from build123d import *

# Parameters (mm, degrees)
BOSS_EXTRUDE1_DEPTH            = 64
BOSS_EXTRUDE2_DEPTH            = 12
SKETCH3_W                      = 12.5
SKETCH3_H                      = 12.5
CUT_EXTRUDE1_DEPTH             = 29
CUT_EXTRUDE2_REACH             = 106.125
SKETCH5_W                      = 12.5
SKETCH5_H                      = 17
CUT_EXTRUDE2_DIRECTION_2_REACH = 106.125
CUT_EXTRUDE3_REACH             = 116.092
SKETCH6_R                      = 2
SKETCH7_W                      = 80
SKETCH7_H                      = 29
BOSS_EXTRUDE3_DEPTH            = 10
SKETCH8_W                      = 5
SKETCH8_H                      = 17
CUT_EXTRUDE4_DEPTH             = 80


with BuildPart() as part:
    # Sketch1 → Boss-Extrude1 (new body)
    with BuildSketch(Plane.XY):
        with BuildLine():
            Line((0, 0), (80, 0))
            Line((80, 0), (80, 5))
            Line((80, 5), (71, 5))
            Line((71, 5), (71, 22))
            Line((71, 22), (80, 22))
            Line((80, 22), (80, 29))
            Line((80, 29), (65, 29))
            ThreePointArc((65, 29), (40, 4), (15, 29))
            Line((15, 29), (0, 29))
            Line((0, 29), (0, 22))
            Line((0, 22), (9, 22))
            Line((9, 22), (9, 5))
            Line((9, 5), (0, 5))
            Line((0, 5), (0, 0))
        make_face()
    extrude(amount=BOSS_EXTRUDE1_DEPTH)

    # Sketch2 → Boss-Extrude2 (add)
    with BuildSketch(Plane.XY.offset(64)):
        with BuildLine():
            Line((60, 29), (80, 29))
            Line((80, 29), (80, 0))
            Line((80, 0), (0, 0))
            Line((0, 0), (0, 29))
            Line((0, 29), (20, 29))
            ThreePointArc((20, 29), (40, 9), (60, 29))
        make_face()
    extrude(amount=BOSS_EXTRUDE2_DEPTH)

    # Sketch3 → Cut-Extrude1 (cut)
    with BuildSketch(Plane(origin=(0, 29, 0), x_dir=(1, 0, 0), z_dir=(0, 1, 0))):
        with Locations((21.25, -16)):
            Rectangle(SKETCH3_W, SKETCH3_H)
        with Locations((58.75, -16)):
            Rectangle(SKETCH3_W, SKETCH3_H)
        with Locations((21.25, -48)):
            Rectangle(SKETCH3_W, SKETCH3_H)
        with Locations((58.75, -48)):
            Rectangle(SKETCH3_W, SKETCH3_H)
    extrude(amount=-CUT_EXTRUDE1_DEPTH, mode=Mode.SUBTRACT)

    # Cut-Extrude2: up to this face of the body (flat: up to its plane)
    cut_extrude2_end = Plane(part.part.faces().sort_by_distance((9, 13.5, 32))[0])
    # Sketch5 → Cut-Extrude2 (cut, up to the picked face)
    with BuildSketch(Plane(origin=(15, 0, 0), x_dir=(0, 0, -1), z_dir=(1, 0, 0)), mode=Mode.PRIVATE) as cut_extrude2_sk1:
        with Locations((-48, 13.5)):
            Rectangle(SKETCH5_W, SKETCH5_H)
    cut_extrude2_tool1 = split(extrude(cut_extrude2_sk1.sketch, amount=-CUT_EXTRUDE2_REACH, mode=Mode.PRIVATE), bisect_by=cut_extrude2_end, keep=Keep.BOTH, mode=Mode.PRIVATE)
    # Sketch5 → Cut-Extrude2 (cut, up to the picked face)
    with BuildSketch(Plane(origin=(15, 0, 0), x_dir=(0, 0, -1), z_dir=(1, 0, 0)), mode=Mode.PRIVATE) as cut_extrude2_sk2:
        with Locations((-16, 13.5)):
            Rectangle(SKETCH5_W, SKETCH5_H)
    cut_extrude2_tool2 = split(extrude(cut_extrude2_sk2.sketch, amount=-CUT_EXTRUDE2_REACH, mode=Mode.PRIVATE), bisect_by=cut_extrude2_end, keep=Keep.BOTH, mode=Mode.PRIVATE)
    add(cut_extrude2_tool1.solids().sort_by(Axis((15, 13.5, 48), (-1, 0, 0)))[0], mode=Mode.SUBTRACT)
    add(cut_extrude2_tool2.solids().sort_by(Axis((15, 13.5, 16), (-1, 0, 0)))[0], mode=Mode.SUBTRACT)

    # Cut-Extrude2 direction 2: up to this face of the body (flat: up to its plane)
    cut_extrude2_direction_2_end = Plane(part.part.faces().sort_by_distance((71, 13.5, 32))[0])
    # Sketch5 → Cut-Extrude2 direction 2 (cut, up to the picked face)
    with BuildSketch(Plane(origin=(15, 0, 0), x_dir=(0, 0, -1), z_dir=(1, 0, 0)), mode=Mode.PRIVATE) as cut_extrude2_direction_2_sk1:
        with Locations((-48, 13.5)):
            Rectangle(SKETCH5_W, SKETCH5_H)
    cut_extrude2_direction_2_tool1 = split(extrude(cut_extrude2_direction_2_sk1.sketch, amount=CUT_EXTRUDE2_DIRECTION_2_REACH, mode=Mode.PRIVATE), bisect_by=cut_extrude2_direction_2_end, keep=Keep.BOTH, mode=Mode.PRIVATE)
    # Sketch5 → Cut-Extrude2 direction 2 (cut, up to the picked face)
    with BuildSketch(Plane(origin=(15, 0, 0), x_dir=(0, 0, -1), z_dir=(1, 0, 0)), mode=Mode.PRIVATE) as cut_extrude2_direction_2_sk2:
        with Locations((-16, 13.5)):
            Rectangle(SKETCH5_W, SKETCH5_H)
    cut_extrude2_direction_2_tool2 = split(extrude(cut_extrude2_direction_2_sk2.sketch, amount=CUT_EXTRUDE2_DIRECTION_2_REACH, mode=Mode.PRIVATE), bisect_by=cut_extrude2_direction_2_end, keep=Keep.BOTH, mode=Mode.PRIVATE)
    add(cut_extrude2_direction_2_tool1.solids().sort_by(Axis((15, 13.5, 48), (1, 0, 0)))[0], mode=Mode.SUBTRACT)
    add(cut_extrude2_direction_2_tool2.solids().sort_by(Axis((15, 13.5, 16), (1, 0, 0)))[0], mode=Mode.SUBTRACT)

    # Cut-Extrude3: up to this face of the body (flat: up to its plane)
    cut_extrude3_end = Plane(part.part.faces().sort_by_distance((72, 29, 39.6))[0])
    # Sketch6 → Cut-Extrude3 (cut, up to the picked face)
    with BuildSketch(Plane(origin=(0, 0, 0), x_dir=(-1, 0, 0), z_dir=(0, -1, 0)), mode=Mode.PRIVATE) as cut_extrude3_sk1:
        with Locations(Location((-4.499910861, -59.125, 0), (0, 0, 90))):
            Circle(SKETCH6_R)
    cut_extrude3_tool1 = split(extrude(cut_extrude3_sk1.sketch, amount=-CUT_EXTRUDE3_REACH, mode=Mode.PRIVATE), bisect_by=cut_extrude3_end, keep=Keep.BOTH, mode=Mode.PRIVATE)
    # Sketch6 → Cut-Extrude3 (cut, up to the picked face)
    with BuildSketch(Plane(origin=(0, 0, 0), x_dir=(-1, 0, 0), z_dir=(0, -1, 0)), mode=Mode.PRIVATE) as cut_extrude3_sk2:
        with Locations(Location((-4.499910861, -4.875, 0), (0, 0, 180))):
            Circle(SKETCH6_R)
    cut_extrude3_tool2 = split(extrude(cut_extrude3_sk2.sketch, amount=-CUT_EXTRUDE3_REACH, mode=Mode.PRIVATE), bisect_by=cut_extrude3_end, keep=Keep.BOTH, mode=Mode.PRIVATE)
    # Sketch6 → Cut-Extrude3 (cut, up to the picked face)
    with BuildSketch(Plane(origin=(0, 0, 0), x_dir=(-1, 0, 0), z_dir=(0, -1, 0)), mode=Mode.PRIVATE) as cut_extrude3_sk3:
        with Locations(Location((-75.500089139, -4.875, 0), (0, 0, 180))):
            Circle(SKETCH6_R)
    cut_extrude3_tool3 = split(extrude(cut_extrude3_sk3.sketch, amount=-CUT_EXTRUDE3_REACH, mode=Mode.PRIVATE), bisect_by=cut_extrude3_end, keep=Keep.BOTH, mode=Mode.PRIVATE)
    # Sketch6 → Cut-Extrude3 (cut, up to the picked face)
    with BuildSketch(Plane(origin=(0, 0, 0), x_dir=(-1, 0, 0), z_dir=(0, -1, 0)), mode=Mode.PRIVATE) as cut_extrude3_sk4:
        with Locations(Location((-75.500089139, -59.125, 0), (0, 0, 180))):
            Circle(SKETCH6_R)
    cut_extrude3_tool4 = split(extrude(cut_extrude3_sk4.sketch, amount=-CUT_EXTRUDE3_REACH, mode=Mode.PRIVATE), bisect_by=cut_extrude3_end, keep=Keep.BOTH, mode=Mode.PRIVATE)
    add(cut_extrude3_tool1.solids().sort_by(Axis((4.499911, 0, 59.125), (0, 1, 0)))[0], mode=Mode.SUBTRACT)
    add(cut_extrude3_tool2.solids().sort_by(Axis((4.499911, 0, 4.875), (0, 1, 0)))[0], mode=Mode.SUBTRACT)
    add(cut_extrude3_tool3.solids().sort_by(Axis((75.500089, 0, 4.875), (0, 1, 0)))[0], mode=Mode.SUBTRACT)
    add(cut_extrude3_tool4.solids().sort_by(Axis((75.500089, 0, 59.125), (0, 1, 0)))[0], mode=Mode.SUBTRACT)

    # Sketch7 → Boss-Extrude3 (add)
    with BuildSketch(Plane(origin=(0, 0, 0), x_dir=(-1, 0, 0), z_dir=(0, 0, -1))):
        with Locations((-40, 14.5)):
            Rectangle(SKETCH7_W, SKETCH7_H)
    extrude(amount=BOSS_EXTRUDE3_DEPTH)

    # Sketch8 → Cut-Extrude4 (cut)
    with BuildSketch(Plane(origin=(80, 0, 0), x_dir=(0, 0, -1), z_dir=(1, 0, 0))):
        with Locations((2.5, 13.5)):
            Rectangle(SKETCH8_W, SKETCH8_H)
    extrude(amount=-CUT_EXTRUDE4_DEPTH, mode=Mode.SUBTRACT)


solid = part.part
Work out the finished part from the listing and answer in its coordinate system (mm). A direction names the side the tool comes from. Give positions to 0.01 mm unless a question says otherwise; leave off trailing zeros. Write each loop counter-clockwise with the first axis right and the second up, starting at its lowest first coordinate (ties: lowest second). Pieces come first, ordered by that corner, then holes.
Q1. The part is cut by section C-C on x = 40. Give the vertices of the cut face in (y, z), and give its area (3 significant figures).
Answer:
outline: (0, -10) - (29, -10) - (29, 0) - (22, 0) - (22, -5) - (5, -5) - (5, 0) - (4, 0) - (4, 64) - (9, 64) - (9, 76) - (0, 76) - close
area: 569 mm2
Q2. The part is cut by section B-B on x = 25.5. Give the vertices of the cut face in (y, z).
Answer:
outline: (0, -10) - (29, -10) - (29, 0) - (22, 0) - (22, -5) - (5, -5) - (5, 0) - (8.63, 0) - (8.63, 9.75) - (0, 9.75) - close; (0, 22.25) - (8.63, 22.25) - (8.63, 41.75) - (0, 41.75) - close; (0, 54.25) - (8.63, 54.25) - (8.63, 64) - (15.23, 64) - (15.23, 76) - (0, 76) - close
Q3. Straight lines are drawn through the part: L1, parallel to Z at x = 15, y = 15.25; L2, parallel to Z at x = 18, y = 3.25; L3, parallel to Y at x = 5, z = 31. For each, find the intervals that lie inside material, in ascending order.
Answer:
L1: z = -10 to -5, 0 to 9.75, 22.25 to 41.75, 54.25 to 76
L2: z = -10 to 9.75, 22.25 to 41.75, 54.25 to 76
L3: y = 0 to 5, 22 to 29
Q4. Given pin 1 (7.5 mm diameter, centred on x = 34.5, y = 26.5, fed in from +Z); pin 2 (8 mm diameter, centred on y = 17.5, z = 25.5, fed in from +X); pin 3 (5 mm diameter, centred on y = 17, z = 7, fed in from -X), each flat-ended and moving along its own axis, determine where each tip first touches the part or whether it passes through.
Answer:
pin 1: stops at z = 0
pin 2: stops at x = 71
pin 3: stops at x = 9
Q5. A tool of negligible diameter and unlimited length cuts with its end or side. For faces 1 (the face through (15, 3, 16)), 2 (the face through (40, 5, -1)), 3 (the face through (71, 13, 5)), 4 (the face through (9, 14, 5)), from which of +Z, -Z, +X, -X, +Y, -Y can it reach the whole face along a straight path? Write none if from no direction.
Answer:
face 1: +Y, -Y
face 2: none
face 3: +X
face 4: -X
Q6. For a pull along Z with two mould halves and no side action, classify faces 5 (the face through (67, 29, 34)), 6 (the face through (65, 11, 0)) as released by +Z, released by -Z, zero draft, split by the parting line, or undercut.
Answer:
face 5: zero draft
face 6: undercut
Q7. The part is cut by section A-A on z = 11. Give the vertices of the cut face in (x, y), and give its area (3 significant figures).
Answer:
outline: (0, 0) - (15, 0) - (15, 5) - (0, 5) - close; (0, 22) - (15, 22) - (15, 29) - (0, 29) - close; (27.5, 0) - (52.5, 0) - (52.5, 5) - (47, 5) arc R25 cw to (33, 5) - (27.5, 5) - close; (65, 0) - (80, 0) - (80, 5) - (65, 5) - close; (65, 22) - (80, 22) - (80, 29) - (65, 29) - close
area: 476 mm2
Q8. The part is cut by section D-D on y = 10.5. State how many separate pieces and enclosed holes the cut face has, and give its area (3 significant figures).
Answer:
separate pieces: 7
enclosed holes: 0
area: 2,280 mm2
